from build123d import *

# Parameters (mm, degrees)
F0_R      = 2.75
F0_R_2    = 10
F1_DEPTH  = 6.35
F3_DEPTH  = 6.35
F4_DEPTH  = 20
F6_DEPTH  = 35
F7_R      = 4.5
F8_DEPTH  = 12.6
F9_R      = 5
F10_R     = 1
F11_DEPTH = 28.65


# Not quite as in the source:
# - a feature names something its author has since deleted; it is built from what else it names


with BuildPart() as f1:
    # F0 (on Top) → F1 (new body)
    with BuildSketch(Plane.XY):
        Polygon((0, 99.6984848098), (-29.6984848098, 70), (-29.6984848098, -10.0008162295), (29.6984848098, -10.0008162295), (29.6984848098, 70), align=None)
        with BuildLine():
            Line((-26.2613506757, -5.0341163975), (-26.3197790794, -0.4248570541))
            ThreePointArc((-26.3197790794, -0.4248570541), (-23.5643542567, 2.3599942046), (-20.8203872227, -0.436147316))
            Line((-20.8203872227, -0.436147316), (-20.892389105, -4.7262623825))
            ThreePointArc((-20.892389105, -4.7262623825), (-23.4159197643, -7.6871530789), (-26.2613506757, -5.0341163975))
        make_face(mode=Mode.SUBTRACT)
        with BuildLine():
            ThreePointArc((-26.32, 46.75), (-23.57, 49.5), (-20.82, 46.75))
            Line((-20.82, 46.75), (-20.82, 42.1391243117))
            ThreePointArc((-20.82, 42.1391243117), (-23.57, 39.3891243117), (-26.32, 42.1391243117))
            Line((-26.32, 42.1391243117), (-26.32, 46.75))
        make_face(mode=Mode.SUBTRACT)
        with BuildLine():
            ThreePointArc((-20, 23.18), (0, 43.18), (20, 23.18))
            Line((20, 23.18), (20, 18.572))
            ThreePointArc((20, 18.572), (0, -1.428), (-20, 18.572))
            Line((-20, 18.572), (-20, 23.18))
        make_face(mode=Mode.SUBTRACT)
        with BuildLine():
            ThreePointArc((20.820000121, -0.3891841763), (23.5802388964, 2.359980939), (26.3199297103, -0.409661849))
            Line((26.3199297103, -0.409661849), (26.290062332, -4.5869490924))
            ThreePointArc((26.290062332, -4.5869490924), (23.7771177689, -7.7443772963), (20.8186322617, -5))
            Line((20.8186322617, -5), (20.820000121, -0.3891841763))
        make_face(mode=Mode.SUBTRACT)
        with BuildLine():
            Line((20.82, 42.1391243117), (20.82, 46.75))
            ThreePointArc((20.82, 46.75), (23.57, 49.5), (26.32, 46.75))
            Line((26.32, 46.75), (26.32, 42.1391243117))
            ThreePointArc((26.32, 42.1391243117), (23.57, 39.3891243117), (20.82, 42.1391243117))
        make_face(mode=Mode.SUBTRACT)
        with Locations((-18.25, 70)):
            Circle(F0_R, mode=Mode.SUBTRACT)
        with Locations((0, 70)):
            Circle(F0_R_2, mode=Mode.SUBTRACT)
        with Locations((18.25, 70)):
            Circle(F0_R, mode=Mode.SUBTRACT)
    extrude(amount=F1_DEPTH)

    # F2 (on Top) → F3 (join)
    with BuildSketch(Plane.XY):
        Polygon((-29.6984848098, 70), (0, 99.6984848098), (0, 112.4264068712), (-46.6550865276, 65.7713203436), (-46.6550865276, 53.0433982822), (-40.3050865276, 59.3933982822), align=None)
        Polygon((-29.6984848098, -10.0008162295), (-29.6984848098, 70), (-40.3050865276, 59.3933982822), (-40.3050865276, -10.0008162295), align=None)
        Polygon((-40.3050865276, -10.0008162295), (-40.3050865276, 59.3933982822), (-46.6550865276, 53.0433982822), (-46.6550865276, -10.0008162295), align=None)
        Polygon((40.3050865276, 59.3933982822), (29.6984848098, 70), (29.6984848098, -10.0008162295), (40.3050865276, -10.0008162295), align=None)
        Polygon((46.6550865276, 53.0433982822), (40.3050865276, 59.3933982822), (40.3050865276, -10.0008162295), (46.6550865276, -10.0008162295), align=None)
        Polygon((0, 112.4264068712), (0, 99.6984848098), (29.6984848098, 70), (40.3050865276, 59.3933982822), (46.6550865276, 53.0433982822), (46.6550865276, 65.7713203436), align=None)
    extrude(amount=F3_DEPTH)

    # F2 (on Top) → F4 (join)
    with BuildSketch(Plane.XY):
        Polygon((46.6550865276, 53.0433982822), (40.3050865276, 59.3933982822), (40.3050865276, -10.0008162295), (46.6550865276, -10.0008162295), align=None)
        Polygon((-40.3050865276, -10.0008162295), (-40.3050865276, 59.3933982822), (-46.6550865276, 53.0433982822), (-46.6550865276, -10.0008162295), align=None)
        Polygon((0, 112.4264068712), (0, 99.6984848098), (29.6984848098, 70), (40.3050865276, 59.3933982822), (46.6550865276, 53.0433982822), (46.6550865276, 65.7713203436), align=None)
        Polygon((-29.6984848098, 70), (0, 99.6984848098), (0, 112.4264068712), (-46.6550865276, 65.7713203436), (-46.6550865276, 53.0433982822), (-40.3050865276, 59.3933982822), align=None)
    extrude(amount=F4_DEPTH)

    # F5 (on face) → F6 (join)
    with BuildSketch(Plane(origin=(0, 0, 0), x_dir=(1, 0, 0), z_dir=(0, 0, -1))):
        Polygon((0, -99.6984848098), (-29.6984848098, -70), (-36.7695526217, -77.0710678119), (-5.8406204336, -108), (0, -113.8406204336), (5.8406204336, -108), (36.7695526217, -77.0710678119), (29.6984848098, -70), align=None)
    extrude(amount=-F6_DEPTH)

    # F9 (call 1 of 7: OpenCascade refuses the feature's edges together)
    f9_edges = [f1.edges().sort_by_distance(p)[0] for p in [
        (33.234019, 73.535534, 35),
        (36.769553, 77.071068, 17.5),
    ]]
    fillet(f9_edges, radius=F9_R)

    # F9#2 (call 2 of 7)
    f9_2_edges = [f1.edges().sort_by_distance(p)[0] for p in [
        (-33.234019, 73.535534, 35),
        (-36.769553, 77.071068, 17.5),
    ]]
    fillet(f9_2_edges, radius=F9_R)

    # F9#3 (call 3 of 7)
    f9_3_edges = [f1.edges().sort_by_distance(p)[0] for p in [
        (43.480087, -10.000816, 20),
    ]]
    fillet(f9_3_edges, radius=F9_R)

    # F9#4 (call 4 of 7)
    f9_4_edges = [f1.edges().sort_by_distance(p)[0] for p in [
        (-43.480087, -10.000816, 20),
    ]]
    fillet(f9_4_edges, radius=F9_R)

    # F9#5 (call 5 of 7)
    f9_5_edges = [f1.edges().sort_by_distance(p)[0] for p in [
        (46.655087, 65.77132, 10),
    ]]
    fillet(f9_5_edges, radius=F9_R)

    # F9#6 (call 6 of 7)
    f9_6_edges = [f1.edges().sort_by_distance(p)[0] for p in [
        (0, 113.84062, 17.5),
    ]]
    fillet(f9_6_edges, radius=F9_R)

    # F9#7 (call 7 of 7)
    f9_7_edges = [f1.edges().sort_by_distance(p)[0] for p in [
        (-46.655087, 65.77132, 10),
    ]]
    fillet(f9_7_edges, radius=F9_R)

    # F10 (on face) → F11 (cut, through all)
    with BuildSketch(Plane.XY.offset(35)):
        with Locations((0, 99.6984848098)):
            Circle(F10_R)
    extrude(amount=-F11_DEPTH, mode=Mode.SUBTRACT)


with BuildPart() as f8:
    # F7 (on face) → F8 (new body)
    with BuildSketch(Plane(origin=(56.9203102168, 56.9203102168, 0), x_dir=(-0.7071067812, 0.7071067812, 0), z_dir=(0.7071067812, 0.7071067812, 0))):
        with Locations((44.9974746831, 21.5)):
            Circle(F7_R)
    extrude(amount=-F8_DEPTH)


with BuildPart() as f12_1:
    # F12: instance of F8
    add(f8.part.mirror(Plane.YZ))


with BuildPart() as f1_1:
    add(f1.part)

    # F13: cut F12_1, F8
    add(f12_1.part, mode=Mode.SUBTRACT)
    add(f8.part, mode=Mode.SUBTRACT)


solid = f1_1.part
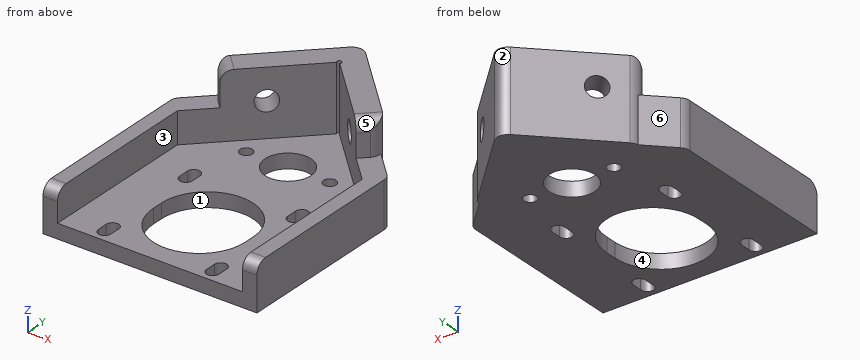
CAD build for the part. Positions are in the model's coordinates, mm. Face numbers are marked on the shaded views. A direction names the side the tool comes from. Coordinates: 2 decimals unless noted, no trailing zeros. Loops run counter-clockwise (first coordinate to the right, second up) from the corner with the lowest first, then second, coordinate; pieces in that order, holes last. Notation, with made-up numbers: (80, 68) - (132, 68) arc R32 cw to (132, 104) - close; hole circle Ø9 at (-25, 77.25). An arc over 180 degrees is marked (long way). Use one line per item in the form item = value. Start each with the question number.
1) Band-saw the part on D-D (x = 18). State how many separate pieces and enclosed holes the cut face has, and give its area (3 significant figures).
2) Band-saw the part on C-C (z = 9.5). Give the cut face in (x, y).
3) Band-saw the part on B-B (x = 6.5). Give the cut face in (y, z), and give its area (3 significant figures).
4) Tool access for the marked faces 1, 2 and 3: list every direction of +Z, -Z, +X, -X, +Y, -Y with a clear straight run to the whole face (end or side of a thin tool).
5) Band-saw the part on A-A (z = 28.5). Give the cut face in (x, y), and give its area (3 significant figures).
6) Flat gauge pins, fed straight in: pin 1 (1 mm diameter, centred on x = 8, z = 31.5, fed in from -Y); pin 2 (18.5 mm diameter, centred on x = -36, y = 28, fed in from +Z); pin 3 (3.5 mm diameter, centred on x = 18.25, y = 70, fed in from -Z); pin 4 (5 mm diameter, centred on y = 99, z = 7, fed in from +X). Where does each tip first touch, or does it go through?
7) Two-plate mould, pull along Y, no slides. Class the marked faces 4, 5 and 6: +Y half, -Y half, draft (parallel to the pull), parting line (faces both ways), or undercut.
8) Drill centre lines: L1, parallel to Y at x = 0, z = 3; L2, parallel to Y at x = -18, z = 5; L3, parallel to Z at x = 38, y = 0. Where is each one in solid material? Low to high. Write a range as from..to.
Check values:
q1.separate_pieces = 3
q1.enclosed_holes = 0
q1.area = 858 mm2
q2.outline = (-46.66, -10) - (-40.31, -10) - (-40.31, 59.39) - (-0.71, 98.99) arc R1 cw (long way) to (0.71, 98.99) - (40.31, 59.39) - (40.31, -10) - (46.66, -10) - (46.66, 63.7) arc R5 ccw to (45.19, 67.24) - (34.65, 77.78) arc R5 ccw to (33.23, 80.61) - (3.54, 110.31) arc R5 ccw to (-3.54, 110.31) - (-33.23, 80.61) arc R5 ccw to (-34.65, 77.78) - (-45.19, 67.24) arc R5 ccw to (-46.66, 63.7) - close
q3.outline = (-10, 0) - (-0.34, 0) - (-0.34, 6.35) - (-10, 6.35) - close; (42.09, 0) - (62.4, 0) - (62.4, 6.35) - (42.09, 6.35) - close; (77.6, 0) - (107.34, 0) - (107.34, 35) - (93.2, 35) - (93.2, 6.35) - (77.6, 6.35) - close
q3.area = 784 mm2
q4.face_1 = +Z, -Z
q4.face_2 = +Z, -Z, +Y
q4.face_3 = +Z, -Y
q5.outline = (-33.23, 73.54) - (-29.7, 70) - (-0.71, 98.99) arc R1 cw (long way) to (0.71, 98.99) - (29.7, 70) - (33.23, 73.54) arc R5 ccw to (33.23, 80.61) - (3.54, 110.31) arc R5 ccw to (-3.54, 110.31) - (-33.23, 80.61) arc R5 ccw to start
q5.area = 922 mm2
q6.pin_1 = 91.2
q6.pin_2 = 20
q6.pin_3 = through
q6.pin_4 = 17.34
q7.face_4 = undercut
q7.face_5 = -Y half
q7.face_6 = +Y half
q8.L1 = -10..-1.43, 43.18..60, 80..111.77
q8.L2 = -10..9.85, 31.9..67.26, 72.74..95.84
q8.L3 = 0..6.35
